```python
from build123d import *

# Parameters (mm, degrees)
SKETCH_1_W          = 50
SKETCH_1_H          = 48
EXTRUDE_1_DEPTH     = 4
FILLET_1_R          = 1
SKETCH_2_R          = 5.25
CUT_EXTRUDE_1_DEPTH = 70.426219831
CUT_EXTRUDE_2_DEPTH = 70.426219831


with BuildPart() as part:
    # 草图1 → 凸台-拉伸1 (new body)
    with BuildSketch(Plane.XY):
        with Locations((25, -24)):
            Rectangle(SKETCH_1_W, SKETCH_1_H)
    extrude(amount=EXTRUDE_1_DEPTH)

    # 圆角1
    fillet_1_edges = [part.edges().sort_by_distance(p)[0] for p in [
        (0, 0, 2),
        (50, 0, 2),
        (50, -48, 2),
        (0, -48, 2),
    ]]
    fillet(fillet_1_edges, radius=FILLET_1_R)

    # 草图2 → 切除-拉伸1 (cut, through all)
    with BuildSketch(Plane.XY.offset(4)):
        with Locations((7.5, -6.5)):
            Circle(SKETCH_2_R)
        with Locations((42.5, -6.5)):
            Circle(SKETCH_2_R)
        with Locations((42.5, -41.5)):
            Circle(SKETCH_2_R)
        with Locations((7.5, -41.5)):
            Circle(SKETCH_2_R)
        with BuildLine():
            Line((25, -24), (29.4, -24))
            ThreePointArc((29.4, -24), (28.111269837, -20.888730163), (25, -19.6))
            Line((25, -19.6), (25, -24))
        make_face()
        with BuildLine():
            Line((20.6, -24), (25, -24))
            Line((25, -24), (25, -19.6))
            ThreePointArc((25, -19.6), (21.888730163, -20.888730163), (20.6, -24))
        make_face()
        with BuildLine():
            ThreePointArc((25, -28.4), (28.111269837, -27.111269837), (29.4, -24))
            Line((29.4, -24), (25, -24))
            Line((25, -24), (25, -28.4))
        make_face()
        with BuildLine():
            Line((25, -28.4), (25, -24))
            Line((25, -24), (20.6, -24))
            ThreePointArc((20.6, -24), (21.888730163, -27.111269837), (25, -28.4))
        make_face()
    extrude(amount=-CUT_EXTRUDE_1_DEPTH, mode=Mode.SUBTRACT)

    # 草图9 → 切除-拉伸2 (cut, through all)
    with BuildSketch(Plane.XY.offset(4)):
        with BuildLine():
            ThreePointArc((4.2, -24), (7.5, -27.3), (10.8, -24))
            Line((10.8, -24), (4.2, -24))
        make_face()
        with BuildLine():
            Line((4.2, -24), (10.8, -24))
            ThreePointArc((10.8, -24), (7.5, -20.7), (4.2, -24))
        make_face()
        with BuildLine():
            ThreePointArc((39.2, -24), (42.5, -27.3), (45.8, -24))
            Line((45.8, -24), (39.2, -24))
        make_face()
        with BuildLine():
            Line((39.2, -24), (45.8, -24))
            ThreePointArc((45.8, -24), (42.5, -20.7), (39.2, -24))
        make_face()
        with BuildLine():
            ThreePointArc((25, -3.2), (21.7, -6.5), (25, -9.8))
            Line((25, -9.8), (25, -3.2))
        make_face()
        with BuildLine():
            Line((25, -3.2), (25, -9.8))
            ThreePointArc((25, -9.8), (27.333452378, -8.833452378), (28.3, -6.5))
            ThreePointArc((28.3, -6.5), (27.333452378, -4.166547622), (25, -3.2))
        make_face()
        with BuildLine():
            ThreePointArc((28.3, -41.5), (27.333452378, -39.166547622), (25, -38.2))
            Line((25, -38.2), (25, -44.8))
            ThreePointArc((25, -44.8), (27.333452378, -43.833452378), (28.3, -41.5))
        make_face()
        with BuildLine():
            Line((25, -44.8), (25, -38.2))
            ThreePointArc((25, -38.2), (21.7, -41.5), (25, -44.8))
        make_face()
    extrude(amount=-CUT_EXTRUDE_2_DEPTH, mode=Mode.SUBTRACT)


solid = part.part
```
Model file for the job. Use its own axes, mm. Coordinates: 2 decimals unless noted, no trailing zeros. Write each loop counter-clockwise with the first axis right and the second up, starting at its lowest first coordinate (ties: lowest second). Pieces come first, ordered by that corner, then holes. Notation, with made-up numbers: (39.25, 20.5) - (67.25, 20.5) arc R17 cw to (67.25, 25.5) - close; hole circle Ø1 at (76.25, 32). An arc over 180 degrees is marked (long way). One line per item, written item: value. Start each with the question number.
1. Mould opens along X. For faces 1 (the flat face through (25, -48, 2)), 2 (the flat face through (50, -24, 2)), 3 (the flat face through (0, -24, 2)), 4 (the cylindrical face through (38.33, -9.69, 2.03)) say: released by +X, released by -X, zero draft, split by the parting line, or undercut.
2. Flat gauge pin, fed straight in: pin 1 (10 mm diameter, centred on x = 12, y = -14.5, fed in from -Z). Where does the tip first touch, or does it go through?
3. Probe line 1 (Y direction, x = 7.5, z = 1.1); line 2 (Y direction, x = 10, z = 0.85); line 3 (X direction, y = -7, z = 3.5). List the from-to ranges inside material, lowest first. Write a range as from..to.
4. Slice it at A-A (x = 7.5). Write the cut outline in (y, z), plus the area to 3 significant figures.
5. Slice it at B-B (z = 1.85). Count the separate pieces of the cut face and the enclosed holes in it, plus the area to 3 significant figures.
6. Slice it at C-C (y = -9). Write the cut outline in (x, z).
Answers below:
1. face 1: zero draft
1. face 2: released by +X
1. face 3: released by -X
1. face 4: undercut
2. pin 1: stops at z = 0
3. line 1: y = -48..-46.75, -36.25..-27.3, -20.7..-11.75, -1.25..0
3. line 2: y = -48..-46.12, -36.88..-26.15, -21.85..-11.12, -1.88..0
3. line 3: x = 0..2.27, 12.73..21.74, 28.26..37.27, 47.73..50
4. outline: (-48, 0) - (-46.75, 0) - (-46.75, 4) - (-48, 4) - close; (-36.25, 0) - (-27.3, 0) - (-27.3, 4) - (-36.25, 4) - close; (-20.7, 0) - (-11.75, 0) - (-11.75, 4) - (-20.7, 4) - close; (-1.25, 0) - (0, 0) - (0, 4) - (-1.25, 4) - close
4. area: 81.6 mm^2
5. separate pieces: 1
5. enclosed holes: 9
5. area: 1,860 mm^2
6. outline: (0, 0) - (2.88, 0) - (2.88, 4) - (0, 4) - close; (12.12, 0) - (22.85, 0) - (22.85, 4) - (12.12, 4) - close; (27.15, 0) - (37.88, 0) - (37.88, 4) - (27.15, 4) - close; (47.12, 0) - (50, 0) - (50, 4) - (47.12, 4) - close
